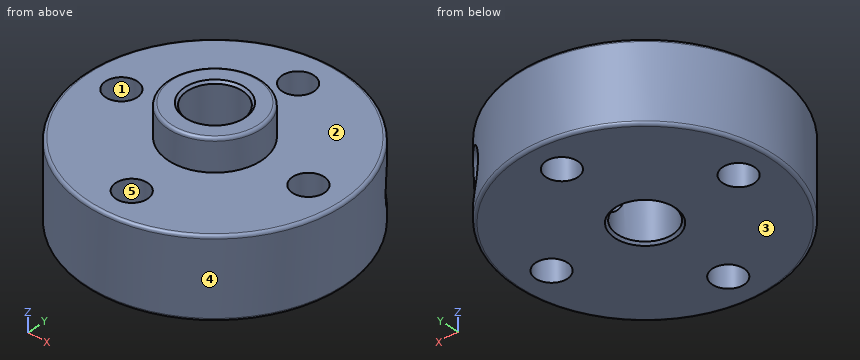
from build123d import *

# Parameters (mm, degrees)
SKETCH1_R           = 11
BOSS_EXTRUDE1_DEPTH = 6.7
SKETCH2_R           = 3.9625
BOSS_EXTRUDE2_DEPTH = 2.7
SKETCH3_R           = 2.365
CUT_EXTRUDE1_DEPTH  = 10.4
SKETCH4_R           = 1.35
CUT_EXTRUDE2_DEPTH  = 7.7
SKETCH6_R           = 2
CUT_EXTRUDE3_DEPTH  = 16.556349186
CHAMFER1_SIZE       = 0.2
FILLET1_R           = 0.25


with BuildPart() as part:
    # Sketch1 → Boss-Extrude1 (new body)
    with BuildSketch(Plane.XY):
        Circle(SKETCH1_R)
    extrude(amount=-BOSS_EXTRUDE1_DEPTH)

    # Sketch2 → Boss-Extrude2 (add)
    with BuildSketch(Plane.XY):
        Circle(SKETCH2_R)
    extrude(amount=BOSS_EXTRUDE2_DEPTH)

    # Sketch3 → Cut-Extrude1 (cut, through all)
    with BuildSketch(Plane.XY.offset(2.7)):
        Circle(SKETCH3_R)
    extrude(amount=-CUT_EXTRUDE1_DEPTH, mode=Mode.SUBTRACT)

    # Sketch4 → Cut-Extrude2 (cut, through all)
    with BuildSketch(Plane.XY):
        with Locations((0, 8)):
            Circle(SKETCH4_R)
        with Locations((8, 0)):
            Circle(SKETCH4_R)
        with Locations((0, -8)):
            Circle(SKETCH4_R)
        with Locations((-8, 0)):
            Circle(SKETCH4_R)
    extrude(amount=-CUT_EXTRUDE2_DEPTH, mode=Mode.SUBTRACT)

    # Sketch6 → Cut-Extrude3 (cut, through all)
    with BuildSketch(Plane(origin=(0, 0, 0), x_dir=(0, 0, 1), z_dir=(-0.707106781, -0.707106781, 0))):
        with Locations((-3.5, 0)):
            Circle(SKETCH6_R)
    extrude(amount=-CUT_EXTRUDE3_DEPTH, mode=Mode.SUBTRACT)

    # Chamfer1
    chamfer1_edges = [part.edges().sort_by_distance(p)[0] for p in [
        (-2.365, 0, -6.7),
        (-2.365, 0, 2.7),
    ]]
    chamfer(chamfer1_edges, length=CHAMFER1_SIZE)

    # Fillet1
    fillet1_edges = [part.edges().sort_by_distance(p)[0] for p in [
        (-11, 0, 0),
        (-11, 0, -6.7),
        (-3.9625, 0, 2.7),
    ]]
    fillet(fillet1_edges, radius=FILLET1_R)


solid = part.part
Part model, mm, in its own coordinate system. Face numbers are marked on the shaded views. A direction names the side the tool comes from. Give positions to 0.01 mm unless a question says otherwise; leave off trailing zeros. Order: outer loops, then holes, each group sorted by start corner. A loop starts at its lowest first (then second) coordinate and runs counter-clockwise, first axis right, second up. Notation, with made-up numbers: (-1.5, 18) - (9.5, 18) arc R24 ccw to (9.5, 36) - close; hole circle Ø7 at (42.5, -7). An arc over 180 degrees is marked (long way). Use a Markdown table: item, result.
1) Probe L1, parallel to X at y = 0.5, z = -3.25; L2, parallel to Z at x = -5.25, y = 5.5; L3, parallel to X at y = 4.25, z = -3. List the from-to ranges inside material, lowest first. Write a range as from..to.
Checked values:
| item | result |
|---|---|
| L1 | -10.99..-9.25, -6.75..-2.31, 3.31..6.75, 9.25..10.99 |
| L2 | -6.7..0 |
| L3 | -10.15..1.51, 6.99..10.15 |
2) 3-axis set-ups, long thin cutter, end or side, ignore diameter. For the marked faces 1 and 2: which of +Z, -Z, +X, -X, +Y, -Y reach the whole face in a straight line?
Checked values:
| item | result |
|---|---|
| face 1 | +Z, -Z |
| face 2 | +Z |
3) Flat gauge pins, fed straight in: P1, Ø3, axis at x = 6.5, y = 5.5, coming from the +Z side; P2, Ø12, axis at x = -5.5, y = -2, coming from the +Z side; P3, Ø1.5, axis at x = 3, z = 0, coming from the -Y side; P4, Ø1.5, axis at y = 1, z = -5.5, coming from the +X side. Where does each tip first touch, or does it go through?
Checked values:
| item | result |
|---|---|
| P1 | z = 0 |
| P2 | z = 2.7 |
| P3 | y = -10.76 |
| P4 | x = 11 |
4) Saw through at B-B on x = 0. Count the separate pieces of the cut face and the enclosed holes in it, plus the area to 3 significant figures.
Checked values:
| item | result |
|---|---|
| separate pieces | 4 |
| enclosed holes | 0 |
| area | 87.3 mm² |
5) Two-plate mould, pull along Y, no slides. Class the marked faces 3, 4 and 5: +Y half, -Y half, draft (parallel to the pull), parting line (faces both ways), or undercut.
Checked values:
| item | result |
|---|---|
| face 3 | draft |
| face 4 | parting line |
| face 5 | undercut |
6) Saw through at A-A on z = -3.75. List the corners of the cut face in (x, y) (3 decimals).
Checked values:
| item | result |
|---|---|
| outline | (-0.493, 2.313) - (6.247, 9.054) arc R11 ccw (long way) to (9.054, 6.247) - (2.313, -0.493) arc R2.365 cw (long way) to start; hole circle Ø2.7 at (-8, 0); hole circle Ø2.7 at (0, -8); hole circle Ø2.7 at (0, 8); hole circle Ø2.7 at (8, 0) |
